Geometry check sheet. Reference: the model listing, model coordinates, mm. Face numbers are marked on the shaded views. A direction names the side the tool comes from. Round coordinates to 2 decimals unless told otherwise and drop trailing zeros. Order: outer loops, then holes, each group sorted by start corner. A loop starts at its lowest first (then second) coordinate and runs counter-clockwise, first axis right, second up.
(1) Cross-section at D-D on y = 46. Enter the section's corners in (x, z) (3 decimals).
(2) Thickness scan on L1, parallel to Y at x = -8, z = 3.1; L2, parallel to Y at x = -3.5, z = 2.7; L3, parallel to X at y = 29, z = 3.65. Record the ranges inside material, lowest first.
(3) Draft check along Y on the marked faces 4, 5 and 6. Enter one of: pulls with the +Y half, pulls with the -Y half, needs draft (parallel to the pull), parting line crosses it, or undercut.
(4) Cross-section at A-A on y = 26. Enter the section's corners in (x, z), and give its area (3 significant figures).
(5) Gauge pin test, flat ends, axial feed: P1, Ø2.5, axis at x = -0.31, y = 10.69, coming from the -Z side; P2, Ø2, axis at y = 46, z = 2.5, coming from the -X side; P3, Ø1.1, axis at x = 1, z = 1.5, coming from the +Y side; P4, Ø1.1, axis at y = 42, z = 1.5, coming from the +X side. Record the tip position at first contact, or that the pin passes through.
(6) Cross-section at C-C on x = -7. Enter the section's corners in (y, z).
(7) Set-up check for the marked faces 1, 2 and 3: record each of +Z, -Z, +X, -X, +Y, -Y from which the full face is reachable in a straight line by a thin tool's end or side.
(8) Cross-section at B-B on x = 14. Enter the section's corners in (y, z), and give its area (3 significant figures).
from build123d import *

# Parameters (mm, degrees)
F1_DEPTH = 3.81
F0_W     = 2.032
F0_H     = 3.81
F2_DEPTH = 1.905
F3_D     = 4


with BuildPart() as f1:
    # F0 (on Top) → F1 (new body)
    with BuildSketch(Plane.XY):
        with BuildLine():
            ThreePointArc((23.2712226898, 27.3948570229), (23.3042181614, 28.1150551719), (23.315220068, 28.8359248085))
            ThreePointArc((23.315220068, 28.8359248085), (19.7805094073, 41.2657152733), (10.234220068, 49.9756079424))
            Line((10.234220068, 49.9756079424), (10.234220068, 48.5526951571))
            Line((10.234220068, 48.5526951571), (12.266220068, 48.5526951571))
            Line((12.266220068, 48.5526951571), (12.266220068, 44.7426951571))
            Line((12.266220068, 44.7426951571), (10.234220068, 44.7426951571))
            Line((10.234220068, 44.7426951571), (10.234220068, 38.0376079424))
            Line((10.234220068, 38.0376079424), (-10.847779932, 38.0376079424))
            Line((-10.847779932, 38.0376079424), (-10.847779932, 44.7426951571))
            Line((-10.847779932, 44.7426951571), (-12.879779932, 44.7426951571))
            Line((-12.879779932, 44.7426951571), (-12.879779932, 48.5526951571))
            Line((-12.879779932, 48.5526951571), (-10.847779932, 48.5526951571))
            Line((-10.847779932, 48.5526951571), (-10.847779932, 49.9756079424))
            ThreePointArc((-10.847779932, 49.9756079424), (-20.7640320202, 40.6469248085), (-23.8847825539, 27.3948570229))
            Line((-23.8847825539, 27.3948570229), (-22.6525039345, 28.1063134155))
            Line((-22.6525039345, 28.1063134155), (-23.6685039345, 29.866077036))
            Line((-23.6685039345, 29.866077036), (-20.3689471461, 31.771077036))
            Line((-20.3689471461, 31.771077036), (-19.3529471461, 30.0113134155))
            Line((-19.3529471461, 30.0113134155), (-13.5461712835, 33.3638570229))
            Line((-13.5461712835, 33.3638570229), (-3.0051712835, 15.1063094603))
            Line((-3.0051712835, 15.1063094603), (-8.8119471461, 11.7537658529))
            Line((-8.8119471461, 11.7537658529), (-7.7959471461, 9.9940022324))
            Line((-7.7959471461, 9.9940022324), (-11.0955039345, 8.0890022324))
            Line((-11.0955039345, 8.0890022324), (-12.1115039345, 9.8487658529))
            Line((-12.1115039345, 9.8487658529), (-13.3437825539, 9.1373094603))
            ThreePointArc((-13.3437825539, 9.1373094603), (-0.306779932, 5.2139248085), (12.7302226898, 9.1373094603))
            Line((12.7302226898, 9.1373094603), (11.4979440704, 9.8487658529))
            Line((11.4979440704, 9.8487658529), (10.4819440704, 8.0890022324))
            Line((10.4819440704, 8.0890022324), (7.182387282, 9.9940022324))
            Line((7.182387282, 9.9940022324), (8.198387282, 11.7537658529))
            Line((8.198387282, 11.7537658529), (2.3916114195, 15.1063094603))
            Line((2.3916114195, 15.1063094603), (12.9326114195, 33.3638570229))
            Line((12.9326114195, 33.3638570229), (18.739387282, 30.0113134155))
            Line((18.739387282, 30.0113134155), (19.755387282, 31.771077036))
            Line((19.755387282, 31.771077036), (23.0549440704, 29.866077036))
            Line((23.0549440704, 29.866077036), (22.0389440704, 28.1063134155))
            Line((22.0389440704, 28.1063134155), (23.2712226898, 27.3948570229))
        make_face()
        Polygon((-7.9324222875, 28.8359248085), (-4.1196011098, 35.4399248085), (3.5060412457, 35.4399248085), (7.3188624234, 28.8359248085), (3.5060412457, 22.2319248085), (-4.1196011098, 22.2319248085), align=None, mode=Mode.SUBTRACT)
    extrude(amount=F1_DEPTH)

    # F0 (on Top) → F2 (join)
    with BuildSketch(Plane.XY):
        with BuildLine():
            ThreePointArc((23.2712226898, 27.3948570229), (23.3042181614, 28.1150551719), (23.315220068, 28.8359248085))
            ThreePointArc((23.315220068, 28.8359248085), (19.7805094073, 41.2657152733), (10.234220068, 49.9756079424))
            Line((10.234220068, 49.9756079424), (10.234220068, 48.5526951571))
            Line((10.234220068, 48.5526951571), (12.266220068, 48.5526951571))
            Line((12.266220068, 48.5526951571), (12.266220068, 44.7426951571))
            Line((12.266220068, 44.7426951571), (10.234220068, 44.7426951571))
            Line((10.234220068, 44.7426951571), (10.234220068, 38.0376079424))
            Line((10.234220068, 38.0376079424), (-10.847779932, 38.0376079424))
            Line((-10.847779932, 38.0376079424), (-10.847779932, 44.7426951571))
            Line((-10.847779932, 44.7426951571), (-12.879779932, 44.7426951571))
            Line((-12.879779932, 44.7426951571), (-12.879779932, 48.5526951571))
            Line((-12.879779932, 48.5526951571), (-10.847779932, 48.5526951571))
            Line((-10.847779932, 48.5526951571), (-10.847779932, 49.9756079424))
            ThreePointArc((-10.847779932, 49.9756079424), (-20.7640320202, 40.6469248085), (-23.8847825539, 27.3948570229))
            Line((-23.8847825539, 27.3948570229), (-22.6525039345, 28.1063134155))
            Line((-22.6525039345, 28.1063134155), (-23.6685039345, 29.866077036))
            Line((-23.6685039345, 29.866077036), (-20.3689471461, 31.771077036))
            Line((-20.3689471461, 31.771077036), (-19.3529471461, 30.0113134155))
            Line((-19.3529471461, 30.0113134155), (-13.5461712835, 33.3638570229))
            Line((-13.5461712835, 33.3638570229), (-3.0051712835, 15.1063094603))
            Line((-3.0051712835, 15.1063094603), (-8.8119471461, 11.7537658529))
            Line((-8.8119471461, 11.7537658529), (-7.7959471461, 9.9940022324))
            Line((-7.7959471461, 9.9940022324), (-11.0955039345, 8.0890022324))
            Line((-11.0955039345, 8.0890022324), (-12.1115039345, 9.8487658529))
            Line((-12.1115039345, 9.8487658529), (-13.3437825539, 9.1373094603))
            ThreePointArc((-13.3437825539, 9.1373094603), (-0.306779932, 5.2139248085), (12.7302226898, 9.1373094603))
            Line((12.7302226898, 9.1373094603), (11.4979440704, 9.8487658529))
            Line((11.4979440704, 9.8487658529), (10.4819440704, 8.0890022324))
            Line((10.4819440704, 8.0890022324), (7.182387282, 9.9940022324))
            Line((7.182387282, 9.9940022324), (8.198387282, 11.7537658529))
            Line((8.198387282, 11.7537658529), (2.3916114195, 15.1063094603))
            Line((2.3916114195, 15.1063094603), (12.9326114195, 33.3638570229))
            Line((12.9326114195, 33.3638570229), (18.739387282, 30.0113134155))
            Line((18.739387282, 30.0113134155), (19.755387282, 31.771077036))
            Line((19.755387282, 31.771077036), (23.0549440704, 29.866077036))
            Line((23.0549440704, 29.866077036), (22.0389440704, 28.1063134155))
            Line((22.0389440704, 28.1063134155), (23.2712226898, 27.3948570229))
        make_face()
        Polygon((-7.9324222875, 28.8359248085), (-4.1196011098, 35.4399248085), (3.5060412457, 35.4399248085), (7.3188624234, 28.8359248085), (3.5060412457, 22.2319248085), (-4.1196011098, 22.2319248085), align=None, mode=Mode.SUBTRACT)
        with Locations((-11.863779932, 46.6476951571)):
            Rectangle(F0_W, F0_H)
        with Locations((11.250220068, 46.6476951571)):
            Rectangle(F0_W, F0_H)
        Polygon((18.739387282, 30.0113134155), (22.0389440704, 28.1063134155), (23.0549440704, 29.866077036), (19.755387282, 31.771077036), align=None)
        Polygon((10.4819440704, 8.0890022324), (11.4979440704, 9.8487658529), (8.198387282, 11.7537658529), (7.182387282, 9.9940022324), align=None)
        Polygon((-8.8119471461, 11.7537658529), (-12.1115039345, 9.8487658529), (-11.0955039345, 8.0890022324), (-7.7959471461, 9.9940022324), align=None)
        Polygon((-23.6685039345, 29.866077036), (-22.6525039345, 28.1063134155), (-19.3529471461, 30.0113134155), (-20.3689471461, 31.771077036), align=None)
    extrude(amount=F2_DEPTH)

    # F3 (through all)
    with Locations(Plane(origin=(0, 0, 0), x_dir=(1, 0, 0), z_dir=(0, 0, -1))):
        with Locations((-16.0198342927, -37.9078609734), (15.4062744286, -37.9078609734), (-0.306779932, -10.6920524787)):
            Hole(F3_D / 2)


solid = f1.part
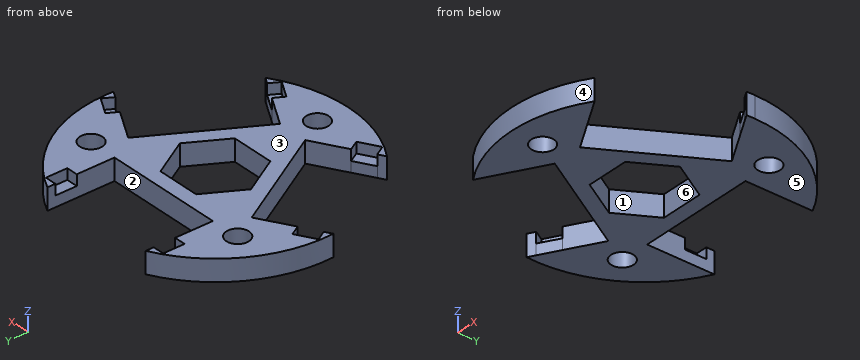
Found:
1. outline: (-16.536, 0) - (-10.848, 0) - (-10.848, 1.905) - (-12.88, 1.905) - (-12.88, 3.81) - (-16.536, 3.81) - close; (10.234, 0) - (15.923, 0) - (15.923, 3.81) - (12.266, 3.81) - (12.266, 1.905) - (10.234, 1.905) - close
2. L1: y = 6.5 to 9.88, 10.35 to 12.22, 23.76 to 38.04
2. L2: y = 5.43 to 14.82, 15.96 to 22.23, 35.44 to 38.04
2. L3: x = -23.93 to -23.17, -11.03 to -7.84, 7.22 to 10.41, 22.55 to 23.31
3. face 4: pulls with the -Y half
3. face 5: needs draft
3. face 6: undercut
4. outline: (-9.29, 0) - (-6.3, 0) - (-6.3, 3.81) - (-9.29, 3.81) - close; (5.68, 0) - (8.68, 0) - (8.68, 3.81) - (5.68, 3.81) - close
4. area: 22.9 mm2
5. P1: passes through
5. P2: stops at x = -17.53
5. P3: stops at y = 38.04
5. P4: stops at x = 19.67
6. outline: (6.18, 0) - (12.8, 0) - (12.8, 3.81) - (6.18, 3.81) - close; (22.03, 0) - (27.22, 0) - (27.22, 3.81) - (22.03, 3.81) - close; (30.45, 0) - (38.04, 0) - (38.04, 3.81) - (30.45, 3.81) - close
7. face 1: +Z, -Z
7. face 2: +Z, -Z, +Y
7. face 3: +Z, +X, -X, +Y, -Y
8. outline: (32.75, 0) - (36.49, 0) - (36.49, 3.81) - (32.75, 3.81) - close; (39.33, 0) - (47.63, 0) - (47.63, 3.81) - (39.33, 3.81) - close
8. area: 45.9 mm2
